Geometry check sheet. Reference: drawing and pictorial views, mm from the part's lowest x, y, z. Coordinates: 2 decimals unless noted, no trailing zeros. Write each loop counter-clockwise with the first axis right and the second up, starting at its lowest first coordinate (ties: lowest second). Pieces come first, ordered by that corner, then holes. Notation, with made-up numbers: (-11.75, 86.25) -> (23.25, 86.25) arc R24 ccw to (23.25, 107.25) -> close; hole circle Ø5 at (-33.5, 39.5). An arc over 180 degrees is marked (long way). Answer in a Markdown table with one row per item.
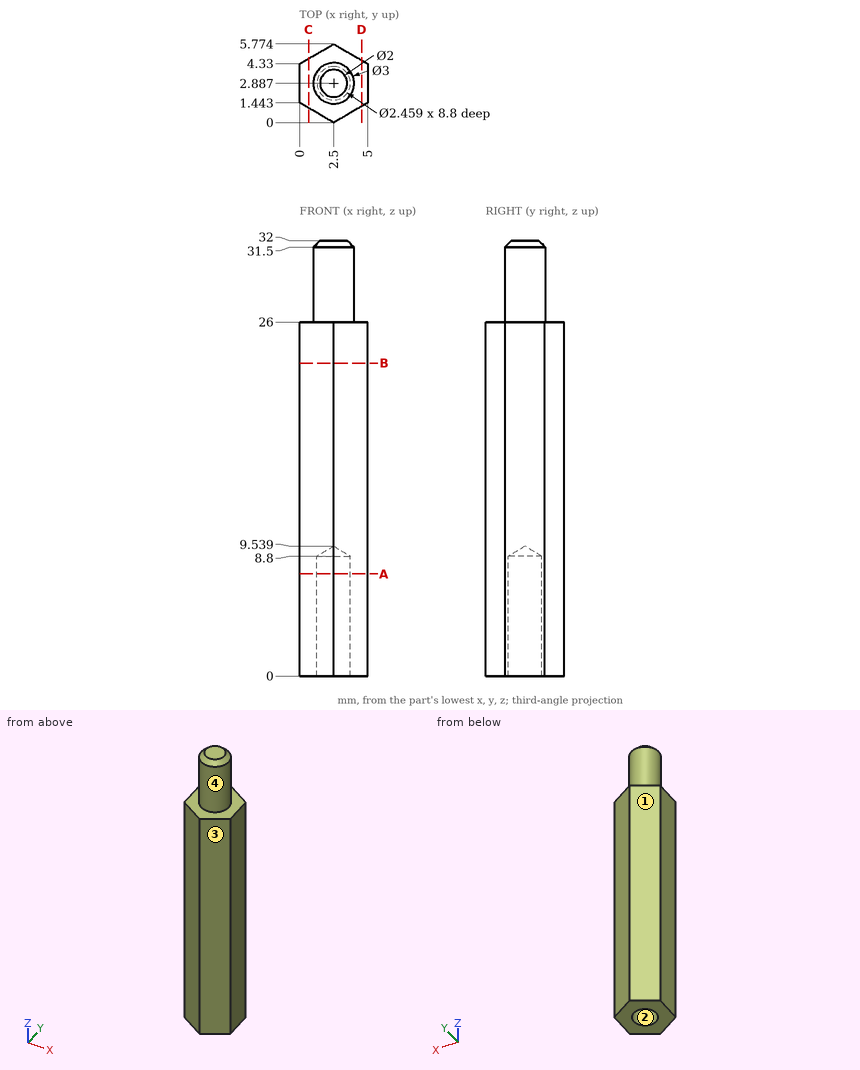
1. Section check C-C, the plane x = 0.65. Record the boundary of the cut face in (y, z) (1 decimal).
Geometry says:
| item | result |
|---|---|
| outline | (1.1, 0) -> (4.7, 0) -> (4.7, 26) -> (1.1, 26) -> close |
2. Section check D-D, the plane x = 4.55. Record the boundary of the cut face in (y, z).
Geometry says:
| item | result |
|---|---|
| outline | (1.18, 0) -> (4.59, 0) -> (4.59, 26) -> (1.18, 26) -> close |
3. Depth check by flat-ended pin: P1, Ø2, axis at x = 0.5, z = 28, coming from the +Y side (1 decimal). Enter the tip coordinate at first touch or a pass-through.
Geometry says:
| item | result |
|---|---|
| P1 | y = 4 |
4. Mould release check, pull along Y, two halves, no side actions. Record for the marked faces 1, 2, 3 and 4: released by +Y, released by -Y, zero draft, split by the parting line, or undercut.
Geometry says:
| item | result |
|---|---|
| face 1 | released by +Y |
| face 2 | undercut |
| face 3 | released by -Y |
| face 4 | split by the parting line |
5. Thickness scan on line 1 (Z direction, x = 2.25, y = 1.15); line 2 (Y direction, x = 2.05, z = 4) (1 decimal); line 3 (Y direction, x = 3.35, z = 7) (1 decimal). Record the ranges inside material, lowest first. Write a range as from..to.
Geometry says:
| item | result |
|---|---|
| line 1 | 0..26 |
| line 2 | 0.3..1.7, 4..5.5 |
| line 3 | 0.5..2, 3.8..5.3 |
6. Section check A-A, the plane z = 7.5. Record the boundary of the cut face in (x, y), plus the area to 3 significant figures.
Geometry says:
| item | result |
|---|---|
| outline | (0, 1.44) -> (2.5, 0) -> (5, 1.44) -> (5, 4.33) -> (2.5, 5.77) -> (0, 4.33) -> close; hole circle Ø2.46 at (2.5, 2.89) |
| area | 16.9 mm^2 |
7. Section check B-B, the plane z = 23. Record the boundary of the cut face in (x, y).
Geometry says:
| item | result |
|---|---|
| outline | (0, 1.44) -> (2.5, 0) -> (5, 1.44) -> (5, 4.33) -> (2.5, 5.77) -> (0, 4.33) -> close |
